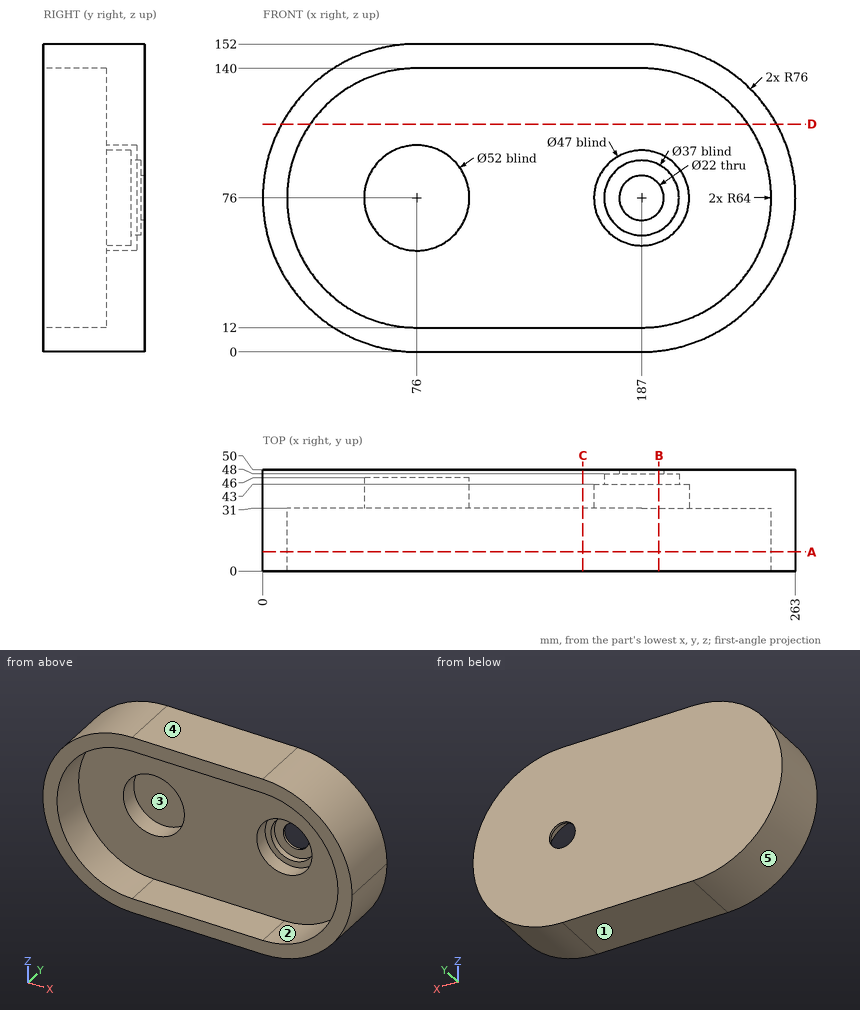
Geometry check sheet. Reference: drawing and pictorial views, mm from the part's lowest x, y, z. A direction names the side the tool comes from. Give positions to 0.01 mm unless a question says otherwise; leave off trailing zeros. Order: outer loops, then holes, each group sorted by start corner. A loop starts at its lowest first (then second) coordinate and runs counter-clockwise, first axis right, second up. Notation, with made-up numbers: M 42,82.5 L 54,82.5 A34 ccw 54,113.5 Z; hole C 75,27.5 d11. An arc over 180 degrees is marked long. Answer in a Markdown table with one row per item. Add a question column.
Q1. Gauge pin test, flat ends, axial feed: pin 1 Ø6 at (x, z) = (131.5, 27) entering from -Y; pin 2 Ø14 at (x, z) = (194.5, 85.5) entering from -Y; pin 3 Ø3 at (x, y) = (51, 26) entering from +Z; pin 4 Ø15.5 at (x, y) = (155.5, 21) entering from -Z. Record the tip position at first contact, or that the pin passes through.
Q2. Sectioned sample at B-B, the plane x = 195.5. Record the boundary of the cut face in (y, z), and give its area (3 significant figures).
Q3. Sectioned sample at C-C, the plane x = 158. Record the boundary of the cut face in (y, z), and give its area (3 significant figures).
Q4. Release check for a two-part mould opening along X. For the marked faces 3, 4 and 5 record: released by +X, released by -X, zero draft, split by the parting line, or undercut.
Q5. Access from +Z, -Z, +X, -X, +Y, -Y to the whole of each face (thin tool, end or side, straight path). Record for the marked faces 1 and 2.
Q6. Sectioned sample at D-D, the plane z = 112.5. Record the boundary of the cut face in (x, y).
Q7. Thickness scan on L1, parallel to Z at x = 163, y = 15; L2, parallel to X at y = 48.9, z = 76; L3, parallel to Z at x = 187, y = 44.2. Record the ranges inside material, lowest first.
Q8. Sectioned sample at A-A, the plane y = 9.5. Record the boundary of the cut face in (x, z), and give its area (3 significant figures).
Verdict:
| question | item | result |
|---|---|---|
| 1 | pin 1 | y = 31 |
| 1 | pin 2 | y = 43 |
| 1 | pin 3 | z = 148.28 |
| 1 | pin 4 | z = 0 |
| 2 | outline | M 0,0.48 L 50,0.48 L 50,69.02 L 48,69.02 L 48,59.57 L 43,59.57 L 43,54.09 L 31,54.09 L 31,12.57 L 0,12.57 Z; M 0,139.43 L 31,139.43 L 31,97.91 L 43,97.91 L 43,92.43 L 48,92.43 L 48,82.98 L 50,82.98 L 50,151.52 L 0,151.52 Z |
| 2 | area | 2,900 mm² |
| 3 | outline | M 0,0 L 50,0 L 50,152 L 0,152 L 0,140 L 31,140 L 31,12 L 0,12 Z |
| 3 | area | 3,630 mm² |
| 4 | face 3 | undercut |
| 4 | face 4 | zero draft |
| 4 | face 5 | released by -X |
| 5 | face 1 | -Z, +X, -X, +Y, -Y |
| 5 | face 2 | -Y |
| 6 | outline | M 9.34,0 L 23.43,0 L 23.43,31 L 239.57,31 L 239.57,0 L 253.66,0 L 253.66,50 L 9.34,50 Z |
| 7 | L1 | 0 to 12, 140 to 152 |
| 7 | L2 | 0 to 176, 198 to 263 |
| 7 | L3 | 0 to 57.5, 94.5 to 152 |
| 8 | outline | M 76,0 L 187,0 A76 ccw 187,152 L 76,152 A76 ccw Z; hole M 76,12 L 187,12 A64 ccw 187,140 L 76,140 A64 ccw Z |
| 8 | area | 7,940 mm² |
